Drawing for the job (mm, zero at the part's lowest x, y, z). Round coordinates to 2 decimals unless told otherwise and drop trailing zeros. Order: outer loops, then holes, each group sorted by start corner. A loop starts at its lowest first (then second) coordinate and runs counter-clockwise, first axis right, second up. Notation, with made-up numbers: (7.25, 21) - (38.25, 21) arc R31 ccw to (38.25, 50) - close; hole circle Ø4 at (34.5, 69). An arc over 180 degrees is marked (long way). Put each result on its own line as item: value. Start each with the question number.
Item 1: Saw through at D-D on y = 153. List the corners of the cut face in (x, z).
Item 2: Saw through at C-C on z = 1.6. List the corners of the cut face in (x, y), plus the area to 3 significant figures.
Item 3: Saw through at B-B on y = 100. List the corners of the cut face in (x, z).
Item 4: Probe probe 1 along X at (y, z) = (100, 2.35); probe 2 along Y at (x, z) = (74.5, 2.7); probe 3 along X at (y, z) = (122.5, 3.9). List the from-to ranges inside material, lowest first.
Item 5: Pin check, flat tips, straight feed: pin 1 Ø1.5 at (y, z) = (107, 1.5) entering from +X; pin 2 Ø2 at (x, y) = (26.5, 90.5) entering from -Z; pin 3 Ø3 at (x, y) = (113.18, 61.82) entering from -Z; pin 4 Ø1 at (y, z) = (106, 1) entering from -X. Stop position of each tip, or through.
Item 6: Saw through at A-A on x = 75. List the corners of the cut face in (y, z), plus the area to 3 significant figures.
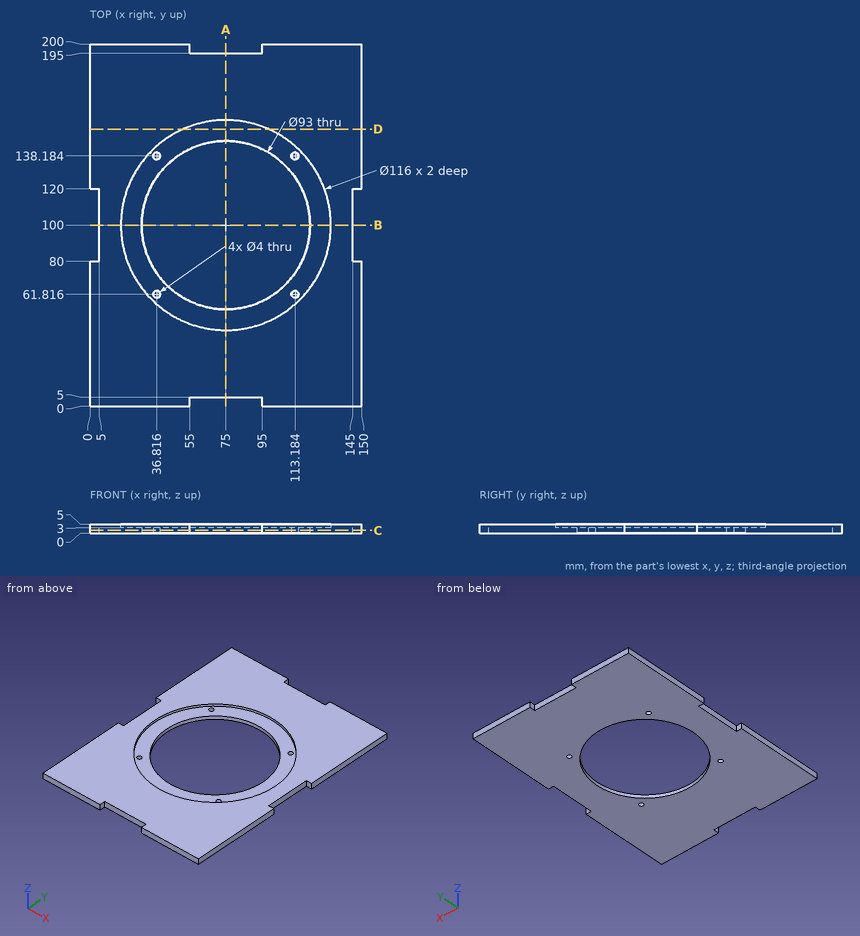
Results found:
1. outline: (0, 0) - (150, 0) - (150, 5) - (98.56, 5) - (98.56, 3) - (51.44, 3) - (51.44, 5) - (0, 5) - close
2. outline: (0, 0) - (55, 0) - (55, 5) - (95, 5) - (95, 0) - (150, 0) - (150, 80) - (145, 80) - (145, 120) - (150, 120) - (150, 200) - (95, 200) - (95, 195) - (55, 195) - (55, 200) - (0, 200) - (0, 120) - (5, 120) - (5, 80) - (0, 80) - close; hole circle Ø93 at (75, 100); hole circle Ø4 at (36.82, 61.82); hole circle Ø4 at (36.82, 138.18); hole circle Ø4 at (113.18, 61.82); hole circle Ø4 at (113.18, 138.18)
2. area: 22,400 mm²
3. outline: (5, 0) - (28.5, 0) - (28.5, 3) - (17, 3) - (17, 5) - (5, 5) - close; (121.5, 0) - (145, 0) - (145, 5) - (133, 5) - (133, 3) - (121.5, 3) - close
4. probe 1: x = 5 to 28.5, 121.5 to 145
4. probe 2: y = 5 to 53.5, 146.5 to 195
4. probe 3: x = 0 to 21.54, 128.46 to 150
5. pin 1: stops at x = 145
5. pin 2: stops at z = 0
5. pin 3: passes through
5. pin 4: stops at x = 5
6. outline: (5, 0) - (53.5, 0) - (53.5, 3) - (42, 3) - (42, 5) - (5, 5) - close; (146.5, 0) - (195, 0) - (195, 5) - (158, 5) - (158, 3) - (146.5, 3) - close
6. area: 439 mm²
